Autodesk Fusion 360 part; units mm, degrees
sketch "Sketch1" plane through (0, 0, 0) normal (0, 0, 1) x (1, 0, 0)
  line L0 (25, 9.5) -> (-25, 9.5)
  line L1 (-25, 9.5) -> (-25, -9.5)
  line L2 (-25, -9.5) -> (25, -9.5)
  line L3 (25, -9.5) -> (25, 9.5)
  line L4 (25, 9.5) -> (-25, -9.5) construction
  line L5 (-25, 9.5) -> (25, -9.5) construction
  line L6 (60, -9.5) -> (110, -9.5)
  line L7 (110, -9.5) -> (110, 9.5)
  line L8 (110, 9.5) -> (60, 9.5)
  line L9 (60, 9.5) -> (60, -9.5)
  line L10 (60, -9.5) -> (110, 9.5) construction
  line L11 (110, -9.5) -> (60, 9.5) construction
  circle A0 centre (75, 0) radius 2
  circle A1 centre (95, 0) radius 2
  point P0 (85, 0)
  dimension "d1" = 50
  dimension "d2" = 19
  dimension "d22" = 50
  dimension "d23" = 19
  dimension "d26" = 4
  dimension "d27" = 4
extrude "Extrude1" add sketch "Sketch1" along normal blind 30 contours L0 L1 L2 L3
sketch "Sketch2" plane through (0, -9.5, 0) normal (0, -1, 0) x (1, 0, 0)
  line L0 (-25, 0) -> (25, 0)
  line L1 (25, 0) -> (25, 30)
  line L2 (25, 30) -> (-25, 30)
  line L3 (-25, 30) -> (-25, 0)
  circle A0 centre (0.0655, 20) radius 14.5
  line L4 (-40, 20) -> (55, 20)
  circle A1 centre (17.5655, 20) radius 2
  circle A2 centre (-17.4345, 20) radius 2
  dimension "d5" = 29
  dimension "d10" = 4
  dimension "d11" = 17.5
  dimension "d12" = 4
  dimension "d13" = 17.5
extrude "Extrude2" cut sketch "Sketch2" against normal blind 19 contours L4 A2 | L4 A2 | L4 A1 | L4 A1 | L2 A0 L4 | A0 L4
sketch "Sketch3" plane through (0, 0, 0) normal (0, 0, -1) x (-1, 0, 0)
  line L0 (-25, 9.5) -> (-25, -9.5)
  line L1 (-25, -9.5) -> (25, -9.5)
  line L2 (25, -9.5) -> (25, 9.5)
  line L3 (25, 9.5) -> (-25, 9.5)
  circle A0 centre (-10, 0) radius 1.5
  circle A1 centre (-10, 0) radius 2.75
  circle A2 centre (10, 0) radius 1.5
  circle A3 centre (10, 0) radius 2.75
  dimension "d14" = 3
  dimension "d15" = 5.5
  dimension "d16" = 3
  dimension "d17" = 5.5
extrude "Extrude3" cut sketch "Sketch3" against normal blind 15 contours A0 | A1 | A2 | A3
extrude "Extrude4" add sketch "Sketch3" against normal blind 3 contours A1 | A3
Part model, mm, in its own coordinate system. A direction names the side the tool comes from. Round coordinates to 2 decimals unless told otherwise and drop trailing zeros. Loops run counter-clockwise (first coordinate to the right, second up) from the corner with the lowest first, then second, coordinate; pieces in that order, holes last.
Item 1: Cut at C-C, the plane x = 10. Give the cut face in (y, z).
Item 2: Drill centre lines: line 1 (X direction, y = 0.75, z = 20); line 2 (X direction, y = 0.5, z = 20.5); line 3 (X direction, y = -4.5, z = 12). Where is each one in solid material? Low to high.
Item 3: Drop flat-ended pins along their axis: P1, Ø17.5, axis at x = 0.07, z = 20, coming from the -Y side; P2, Ø2.5, axis at x = -10, y = 0, coming from the -Z side. Give the stop position or say it passes through.
Item 4: 3-axis set-ups, long thin cutter, end or side, ignore diameter. For faces 4 (the face through (-12.62, 0.83, 6.9)), 5 (the face through (11.5, 0.07, 1.48)), 6 (the face through (-17.695, -0.133, 21.983)): which of +Z, -Z, +X, -X, +Y, -Y reach the whole face in a straight line?
Item 5: Cut at B-B, the plane y = 7.5. Give the cut face in (x, z).
Item 6: Mould opens along X. For faces 1 (the face through (17.305, -0.133, 21.983)), 2 (the face through (-25, 0, 15)), 3 (the face through (0, -9.5, 5)) say: +X half, -X half, draft (parallel to the pull), parting line (faces both ways), or undercut.
Item 7: Cut at A-A, the plane z = 20. Give the cut face in (x, y), then the cut area to 3 significant figures.
Item 8: Cut at D-D, the plane y = 0. Give the cut face in (x, z).
A:
1. outline: (-9.5, 0) - (-1.5, 0) - (-1.5, 3) - (-2.75, 3) - (-2.75, 9.44) - (-9.5, 9.44) - close; (1.5, 0) - (9.5, 0) - (9.5, 9.44) - (2.75, 9.44) - (2.75, 3) - (1.5, 3) - close
2. line 1: x = -25 to -19.43, -15.43 to -14.43, 14.57 to 15.57, 19.57 to 25
2. line 2: x = -25 to -19.37, -15.5 to -14.43, 14.56 to 15.63, 19.5 to 25
2. line 3: x = -25 to -12.03, 12.16 to 25
3. P1: passes through
3. P2: stops at z = 29.07
4. face 4: none
4. face 5: -Z
4. face 6: +Y, -Y
5. outline: (-25, 0) - (25, 0) - (25, 30) - (10.57, 30) arc R14.5 cw (long way) to (-10.43, 30) - (-25, 30) - close; hole circle Ø4 at (-17.43, 20); hole circle Ø4 at (17.57, 20)
6. face 1: undercut
6. face 2: -X half
6. face 3: draft
7. outline: (-25, -9.5) - (-19.43, -9.5) - (-19.43, 9.5) - (-25, 9.5) - close; (-15.43, -9.5) - (-14.43, -9.5) - (-14.43, 9.5) - (-15.43, 9.5) - close; (14.57, -9.5) - (15.57, -9.5) - (15.57, 9.5) - (14.57, 9.5) - close; (19.57, -9.5) - (25, -9.5) - (25, 9.5) - (19.57, 9.5) - close
7. area: 247 mm2
8. outline: (-25, 0) - (-11.5, 0) - (-11.5, 3) - (-12.75, 3) - (-12.75, 13.22) arc R14.5 cw to (-10.43, 30) - (-25, 30) - close; (-8.5, 0) - (8.5, 0) - (8.5, 3) - (7.25, 3) - (7.25, 7.41) arc R14.5 cw to (-7.25, 7.48) - (-7.25, 3) - (-8.5, 3) - close; (10.57, 30) arc R14.5 cw to (12.75, 12.97) - (12.75, 3) - (11.5, 3) - (11.5, 0) - (25, 0) - (25, 30) - close; hole circle Ø4 at (-17.43, 20); hole circle Ø4 at (17.57, 20)
